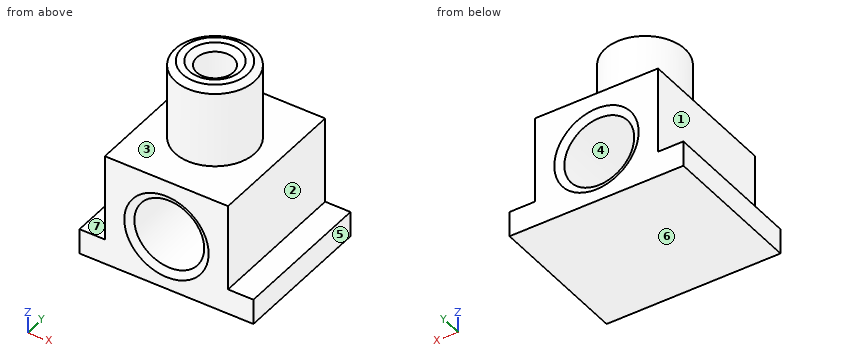
Solid Edge part; units mm, degrees
sketch "Sketch1" plane through (0, 0, 0) normal (0, 0, 1) x (1, 0, 0)
  line L0 (24, -20) -> (24, 20)
  line L1 (24, 20) -> (-24, 20)
  line L2 (-24, 20) -> (-24, -20)
  line L3 (-24, -20) -> (24, -20)
extrude "Protrusion1" add sketch "Sketch1" against normal blind 7
sketch "Sketch2" plane through (0, 0, 0) normal (0, 0, 1) x (1, 0, 0)
  line L0 (17, -20) -> (17, 20)
  line L1 (17, 20) -> (-17, 20)
  line L2 (-17, 20) -> (-17, -20)
  line L3 (-17, -20) -> (17, -20)
extrude "拉伸_2" add sketch "Sketch2" along normal blind 24
sketch "Sketch3" plane through (0, 0, 24) normal (0, 0, 1) x (1, 0, 0)
  circle A0 centre (0, 0) radius 11
extrude "拉伸_3" add sketch "Sketch3" along normal blind 22
hole "孔_1" at (0, 0, 46) direction (0, 0, -1) diameter 10.106 depth 22 tip angle 118 thread major 12 thread length 16
hole "孔_3" at (0, -20, 8) direction (0, 1, 0) diameter 19.294 end up to next
chamfer "倒斜角_2" distance 2 angle 30 4 edges at (-11, 0, 46) (0, 5.053, 46) (-9.647, -20, 8) (0, 20, -1.647) measured on face at (-7.5533, -7.1133, 46) measured on face at (16.48, 20, -1.5233) measured on face at (-16.48, -20, -1.5233)
properties material "钢铁"
CAD build for the part. Positions are in the model's coordinates, mm. Face numbers are marked on the shaded views. A direction names the side the tool comes from. Round coordinates to 2 decimals unless told otherwise and drop trailing zeros. Write each loop counter-clockwise with the first axis right and the second up, starting at its lowest first coordinate (ties: lowest second). Pieces come first, ordered by that corner, then holes.
(1) Slice it at A-A, the plane z = 8. Write the cut outline in (x, y), and give its area (3 significant figures).
(2) Slice it at B-B, the plane y = -17. Write the cut outline in (x, z).
(3) 3-axis set-ups, long thin cutter, end or side, ignore diameter. For the marked faces 1, 2 and 3: which of +Z, -Z, +X, -X, +Y, -Y reach the whole face in a straight line?
(4) Mould opens along Z. For the marked faces 4, 5, 6 and 7 say: pulls with the +Z half, pulls with the -Z half, needs draft (parallel to the pull), parting line crosses it, or undercut.
(5) Probe line 1 along X through (y, z) = (17, 8.5); line 2 along Z through (x, y) = (-14.5, -11.5); line 3 along Z through (x, y) = (5, -13). List the from-to ranges inside material, lowest first.
(6) Slice it at D-D, the plane x = -15. Write the cut outline in (y, z).
(7) Slice it at C-C, the plane z = 26.5. Write the cut outline in (x, y).
(8) Drop flat-ended pins along their axis: P1, Ø12, axis at y = 3, z = 38.5, coming from the -X side; P2, Ø10, axis at x = -5, y = -9.5, coming from the +Z side; P3, Ø7.5, axis at x = 21.5, y = 3, coming from the +Z side; P4, Ø4, axis at y = 9.5, z = 5, coming from the -X side. Give the stop position or say it passes through.
From the geometry:
1. outline: (-17, -20) - (-11.65, -20) - (-9.65, -18.85) - (-9.65, 18.85) - (-11.65, 20) - (-17, 20) - close; (9.65, -18.85) - (11.65, -20) - (17, -20) - (17, 20) - (11.65, 20) - (9.65, 18.85) - close
1. area: 584 mm2
2. outline: (-24, -7) - (24, -7) - (24, 0) - (17, 0) - (17, 24) - (-17, 24) - (-17, 0) - (-24, 0) - close; hole circle Ø19.29 at (0, 8)
3. face 1: +Z, -X, +Y, -Y
3. face 2: +Z, +X, +Y, -Y
3. face 3: +Z
4. face 4: undercut
4. face 5: needs draft
4. face 6: pulls with the -Z half
4. face 7: pulls with the +Z half
5. line 1: x = -17 to -9.63, 9.63 to 17
5. line 2: z = -7 to 24
5. line 3: z = -7 to -0.25, 16.25 to 24
6. outline: (-20, -7) - (20, -7) - (20, 24) - (-20, 24) - close
7. outline: circle Ø22 at (0, 0); hole circle Ø10.11 at (0, 0)
8. P1: stops at x = -11
8. P2: stops at z = 46
8. P3: stops at z = 0
8. P4: stops at x = -17
